from build123d import *

# Parameters (mm, degrees)
SKETCH7_R           = 17.4625
BOSS_EXTRUDE1_DEPTH = 28.56738
CUT_EXTRUDE1_START  = -28.575
CUT_EXTRUDE1_DEPTH  = 28.575
SKETCH10_R          = 4.76885
CUT_EXTRUDE2_DEPTH  = 45.012831156
SKETCH11_R          = 7.2009
CUT_EXTRUDE3_DEPTH  = 1.5875
SKETCH12_R          = 7.9375
CUT_EXTRUDE4_DEPTH  = 37.401344842
CHAMFER2_SIZE       = 1.524


with BuildPart() as part:
    # Sketch7 → Boss-Extrude1 (new body)
    with BuildSketch(Plane.XY):
        Circle(SKETCH7_R)
    extrude(amount=BOSS_EXTRUDE1_DEPTH)

    # Sketch9 → Cut-Extrude1 (cut)
    with BuildSketch(Plane.XY.offset(28.56738).offset(CUT_EXTRUDE1_START)):
        with BuildLine():
            ThreePointArc((10.045651111, 14.28369), (0, 17.4625), (-10.04565111, 14.28369))
            Line((-10.04565111, 14.28369), (10.045651111, 14.28369))
        make_face()
        with BuildLine():
            Line((10.045651111, -14.28369), (-10.04565111, -14.28369))
            ThreePointArc((-10.04565111, -14.28369), (0, -17.4625), (10.045651111, -14.28369))
        make_face()
    extrude(amount=CUT_EXTRUDE1_DEPTH, mode=Mode.SUBTRACT)

    # Sketch10 → Cut-Extrude2 (cut, through all)
    with BuildSketch(Plane(origin=(0, 14.28369, 0), x_dir=(1, 0, 0), z_dir=(0, 1, 0))):
        with Locations(Location((0, -14.28369, 0), (0, 0, 270))):
            Circle(SKETCH10_R)
    extrude(amount=-CUT_EXTRUDE2_DEPTH, mode=Mode.SUBTRACT)

    # Sketch11 → Cut-Extrude3 (cut)
    with BuildSketch(Plane(origin=(0, 14.28369, 0), x_dir=(1, 0, 0), z_dir=(0, 1, 0))):
        with Locations(Location((0, -14.28369, 0), (0, 0, 270))):
            Circle(SKETCH11_R)
    extrude(amount=-CUT_EXTRUDE3_DEPTH, mode=Mode.SUBTRACT)

    # Sketch12 → Cut-Extrude4 (cut, through all)
    with BuildSketch(Plane.XY.offset(28.56738)):
        Circle(SKETCH12_R)
    extrude(amount=-CUT_EXTRUDE4_DEPTH, mode=Mode.SUBTRACT)

    # Chamfer2
    chamfer2_edges = [part.edges().sort_by_distance(p)[0] for p in [
        (17.4625, 0, 0),
        (17.4625, 0, 28.56738),
        (-17.4625, 0, 0),
        (-17.4625, 0, 28.56738),
    ]]
    chamfer(chamfer2_edges, length=CHAMFER2_SIZE)


solid = part.part
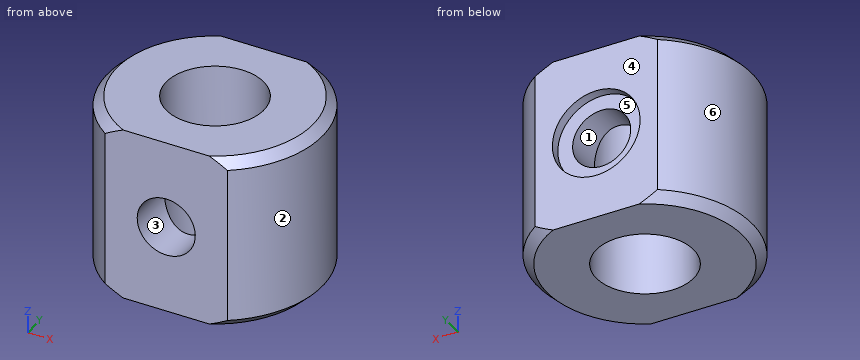
Source: CAD feature listing. Evaluate the final solid. Frame: model axes, mm. Face numbers are marked on the shaded views. A direction names the side the tool comes from. Give positions to 0.01 mm unless a question says otherwise; leave off trailing zeros. Order: outer loops, then holes, each group sorted by start corner. A loop starts at its lowest first (then second) coordinate and runs counter-clockwise, first axis right, second up. Notation, with made-up numbers: (52.25, 67) -> (94.25, 67) arc R32 cw to (94.25, 95) -> close; hole circle Ø3 at (78.5, 9). An arc over 180 degrees is marked (long way). Use a Markdown table: item, result.
1) Section query B-B, the plane x = 0. Return the cut outline in (y, z), then the cut area to 3 significant figures.
Answer list:
| item | result |
|---|---|
| outline | (-14.28, 0) -> (-7.94, 0) -> (-7.94, 9.51) -> (-14.28, 9.51) -> close; (-14.28, 19.05) -> (-7.94, 19.05) -> (-7.94, 28.57) -> (-14.28, 28.57) -> close; (7.94, 0) -> (14.28, 0) -> (14.28, 7.08) -> (12.7, 7.08) -> (12.7, 9.51) -> (7.94, 9.51) -> close; (7.94, 19.05) -> (12.7, 19.05) -> (12.7, 21.48) -> (14.28, 21.48) -> (14.28, 28.57) -> (7.94, 28.57) -> close |
| area | 234 mm² |
2) Reachability of the marked faces 5 and 6 from +Z, -Z, +X, -X, +Y, -Y: full face, straight path, thin tool, end or side. Return the list, or none.
Answer list:
| item | result |
|---|---|
| face 5 | +Y |
| face 6 | +Z, -Z, -X |
3) Contact query for flat-ended pins moving along their axis: P1, Ø7, axis at x = -1.5, z = 15.5, coming from the +Y side; P2, Ø10, axis at y = -10.5, z = 8.5, coming from the -X side; P3, Ø5, axis at y = -4, z = 14.5, coming from the -X side. Output: stop coordinate, or through.
Answer list:
| item | result |
|---|---|
| P1 | y = 12.7 |
| P2 | x = -16.57 |
| P3 | x = -17.4 |
4) Ray query, line 1 along Z through (x, y) = (0, -10.5); line 2 along X through (y, z) = (-2.5, 5.5); line 3 along X through (y, z) = (6.75, 21). Return the intervals inside material, ascending. Write a range as [from, to].
Answer list:
| item | result |
|---|---|
| line 1 | [0, 9.51], [19.05, 28.57] |
| line 2 | [-17.28, -7.53], [7.53, 17.28] |
| line 3 | [-16.11, -4.18], [4.18, 16.11] |
5) Section query A-A, the plane y = 0. Return the cut outline in (x, z), then the cut area to 3 significant figures.
Answer list:
| item | result |
|---|---|
| outline | (-17.46, 1.52) -> (-15.94, 0) -> (-7.94, 0) -> (-7.94, 28.57) -> (-15.94, 28.57) -> (-17.46, 27.04) -> close; (7.94, 0) -> (15.94, 0) -> (17.46, 1.52) -> (17.46, 27.04) -> (15.94, 28.57) -> (7.94, 28.57) -> close |
| area | 540 mm² |
6) Mould query, pull axis X, two halves, no side actions, for the marked faces 1, 2, 3 and 4. Classes: +X half, -X half, draft (parallel to the pull), parting line (faces both ways), or undercut.
Answer list:
| item | result |
|---|---|
| face 1 | undercut |
| face 2 | +X half |
| face 3 | undercut |
| face 4 | draft |
7) Section query C-C, the plane z = 25. Return the cut outline in (x, y) (1 decimal), then the cut area to 3 significant figures.
Answer list:
| item | result |
|---|---|
| outline | (-10, -14.3) -> (10, -14.3) arc R17.5 ccw to (10, 14.3) -> (-10, 14.3) arc R17.5 ccw to start; hole circle Ø15.9 at (0, 0) |
| area | 673 mm² |
8) Section query D-D, the plane x = 6. Return the cut outline in (y, z).
Answer list:
| item | result |
|---|---|
| outline | (-14.28, 0) -> (-5.2, 0) -> (-5.2, 28.57) -> (-14.28, 28.57) -> close; (5.2, 0) -> (14.28, 0) -> (14.28, 10.3) -> (12.7, 10.3) -> (12.7, 18.27) -> (14.28, 18.27) -> (14.28, 28.57) -> (5.2, 28.57) -> close |
